Input: part model. Units: mm. Frame: model coordinates. A direction names the side the tool comes from. Give positions to 0.01 mm unless a question says otherwise; leave off trailing zeros. Write each loop counter-clockwise with the first axis right and the second up, starting at its lowest first coordinate (ties: lowest second). Pieces come first, ordered by that corner, then holes. Notation, with made-up numbers: (27, 17.5) -> (65, 17.5) arc R16 cw to (65, 44.5) -> close; hole circle Ø8 at (-18, -39). An arc over 180 degrees is marked (long way). Return JSON: item names as keys, results as strings. Group by question number.
Item 1: Section A-A, the plane x = 34.5. Return loops of the section in (y, z), then the cut area to 3 significant figures.
Item 2: Line query: line 1 (Y direction, x = 45, z = 3.25); line 2 (X direction, y = 21.5, z = 5.5); line 3 (Z direction, x = 30, y = 9). Output: solid intervals per line, ascending. Write a range as [from, to].
Item 3: Section C-C, the plane y = 7.5. Return loops of the section in (x, z), then the cut area to 3 significant figures.
Item 4: Section B-B, the plane z = 11.25. Return loops of the section in (x, y).
Item 5: Mould query, pull axis X, two halves, no side actions, for faces 6 (the face through (65, 34, 16)), 7 (the face through (76, 75, 3)), 8 (the face through (152, 43, 7)). Classes: released by +X, released by -X, zero draft, split by the parting line, or undercut.
Item 6: Section D-D, the plane x = 107. Return loops of the section in (y, z), then the cut area to 3 significant figures.
Item 7: Pin query (flat end, axial travel): P1, Ø2, axis at x = 45, y = 7.5, coming from the +Z side; P2, Ø21.5, axis at x = 45.5, y = 56, coming from the +Z side; P3, Ø5, axis at x = 106, z = 8, coming from the +Y side; P4, Ø3, axis at x = 149.5, z = 11, coming from the +Y side. Return the tip coordinate at first contact, or that it passes through.
Item 8: Set-up query: faces 1 (the face through (147, 26, 9)), 2 (the face through (150, 43, 10)), 3 (the face through (149.535, 24.523, 12.067)), 4 (the face through (150.4, 55, 12.9)), 5 (the face through (142.2, 39.7, 17)). Return all of +Z, -Z, +X, -X, +Y, -Y with unobstructed straight access to the full face (end or side cutting, diameter ignored); none if empty.
from build123d import *

# Parameters (mm, degrees)
SKETCH1_W           = 152
SKETCH1_H           = 75
SKETCH1_R           = 1.65
BOSS_EXTRUDE1_DEPTH = 5
FILLET1_R           = 10
BOSS_EXTRUDE2_DEPTH = 11
BOSS_EXTRUDE3_DEPTH = 2
CHAMFER1_SIZE       = 7.5
BOSS_EXTRUDE4_DEPTH = 5
FILLET2_R           = 3
SKETCH5_W           = 55
SKETCH5_H           = 8
CUT_EXTRUDE1_DEPTH  = 10


with BuildPart() as part:
    # Sketch1 → Boss-Extrude1 (new body)
    with BuildSketch(Plane.XY):
        with Locations((76, 37.5)):
            Rectangle(SKETCH1_W, SKETCH1_H)
        with Locations((45, 7.5)):
            Circle(SKETCH1_R, mode=Mode.SUBTRACT)
        with Locations((107, 7.5)):
            Circle(SKETCH1_R, mode=Mode.SUBTRACT)
    extrude(amount=BOSS_EXTRUDE1_DEPTH)

    # Fillet1
    fillet1_edges = [part.edges().sort_by_distance(p)[0] for p in [
        (152, 0, 2.5),
        (0, 0, 2.5),
    ]]
    fillet(fillet1_edges, radius=FILLET1_R)

    # Sketch2 → Boss-Extrude2 (add)
    with BuildSketch(Plane.XY.offset(5)):
        Polygon((0, 75), (2, 75), (2, 73), (2, 32), (150, 32), (150, 55), (152, 55), (152, 30), (0, 30), align=None)
    extrude(amount=BOSS_EXTRUDE2_DEPTH)

    # Sketch3 → Boss-Extrude3 (add)
    with BuildSketch(Plane.XY.offset(16)):
        Polygon((152, 30), (152, 55), (146, 55), (146, 36), (6, 36), (6, 75), (0, 75), (0, 30), align=None)
    extrude(amount=BOSS_EXTRUDE3_DEPTH)

    # Chamfer1
    chamfer1_edges = [part.edges().sort_by_distance(p)[0] for p in [
        (146, 36, 17),
    ]]
    chamfer(chamfer1_edges, length=CHAMFER1_SIZE)

    # Sketch4 → Boss-Extrude4 (add)
    with BuildSketch(Plane.ZY):
        Polygon((18, 30), (5, 18), (5, 30), align=None)
    boss_extrude4 = extrude(amount=-BOSS_EXTRUDE4_DEPTH)

    # Mirror1: Boss-Extrude4 across plane
    add(boss_extrude4.mirror(Plane.ZY.offset(-76)))

    # Fillet2
    fillet2_edges = [part.edges().sort_by_distance(p)[0] for p in [
        (149.5, 18, 5),
        (76, 30, 5),
        (2.5, 18, 5),
    ]]
    fillet(fillet2_edges, radius=FILLET2_R)

    # Sketch5 → Cut-Extrude1 (cut)
    with BuildSketch(Plane(origin=(0, 32, 0), x_dir=(1, 0, 0), z_dir=(0, 1, 0))):
        with Locations((39.241088115, -10.5)):
            Rectangle(SKETCH5_W, SKETCH5_H)
    extrude(amount=-CUT_EXTRUDE1_DEPTH, mode=Mode.SUBTRACT)


solid = part.part
Answer below:
{
 "1": {"outline": "(0, 0) -> (75, 0) -> (75, 5) -> (32, 5) -> (32, 6.5) -> (29.6, 6.5) arc R3 cw to (27, 5) -> (0, 5) -> close; (30, 14.5) -> (32, 14.5) -> (32, 16) -> (36, 16) -> (36, 18) -> (30, 18) -> close", "area": "395 mm2"},
 "2": {"line 1": "y = [0, 5.85], [9.15, 75]", "line 2": "x = [0, 5], [147, 152]", "line 3": "z = [0, 5]"},
 "3": {"outline": "(0.32, 0) -> (43.35, 0) -> (43.35, 5) -> (0.32, 5) -> close; (46.65, 0) -> (105.35, 0) -> (105.35, 5) -> (46.65, 5) -> close; (108.65, 0) -> (151.68, 0) -> (151.68, 5) -> (108.65, 5) -> close", "area": "724 mm2"},
 "4": {"outline": "(0, 23.77) -> (5, 23.77) -> (5, 30) -> (11.74, 30) -> (11.74, 32) -> (2, 32) -> (2, 75) -> (0, 75) -> close; (66.74, 30) -> (147, 30) -> (147, 23.77) -> (152, 23.77) -> (152, 55) -> (150, 55) -> (150, 32) -> (66.74, 32) -> close"},
 "5": {"face 6": "undercut", "face 7": "zero draft", "face 8": "released by +X"},
 "6": {"outline": "(0, 0) -> (5.85, 0) -> (5.85, 5) -> (0, 5) -> close; (9.15, 0) -> (75, 0) -> (75, 5) -> (32, 5) -> (32, 16) -> (36, 16) -> (36, 18) -> (30, 18) -> (30, 8) arc R3 cw to (27, 5) -> (9.15, 5) -> close", "area": "394 mm2"},
 "7": {"P1": "passes through", "P2": "stops at z = 5", "P3": "stops at y = 32", "P4": "stops at y = 55"},
 "8": {"face 1": "+Z, -Y", "face 2": "+Y", "face 3": "+Z, +X, -X, -Y", "face 4": "+Z, +X, +Y", "face 5": "+Z, +Y"}
}
